from build123d import *

# Parameters (mm, degrees)
SKETCH_2_R          = 37.505158637
SKETCH_2_R_2        = 2.3
EXTRUDE_2_DEPTH     = 8
SKETCH_3_R          = 33
CUT_EXTRUDE_1_DEPTH = 5
CUT_EXTRUDE_START   = -16
SKETCH_3_2_R        = 33
CUT_EXTRUDE_2_DEPTH = 5


with BuildPart() as part:
    # Sketch 1 → Revolve 1 (revolve)
    with BuildSketch(Plane(origin=(0, 0, 0), x_dir=(0, 0, -1), z_dir=(1, 0, 0))):
        with BuildLine():
            Line((-8, 37.505158637), (8, 37.505158637))
            Line((8, 37.505158637), (10, 41.082575695))
            ThreePointArc((10, 41.082575695), (0, 47.5), (-10, 41.082575695))
            Line((-10, 41.082575695), (-8, 37.505158637))
        make_face()
    revolve(axis=Axis((0, 0, 15.4), (0, 0, -1)))

    # Sketch 2 → Extrude 2 (add, symmetric)
    with BuildSketch(Plane.XY):
        Circle(SKETCH_2_R)
        Circle(SKETCH_2_R_2, mode=Mode.SUBTRACT)
        with Locations((0, 8)):
            Circle(SKETCH_2_R_2, mode=Mode.SUBTRACT)
        with Locations((6.92820323, 4)):
            Circle(SKETCH_2_R_2, mode=Mode.SUBTRACT)
        with Locations((6.92820323, -4)):
            Circle(SKETCH_2_R_2, mode=Mode.SUBTRACT)
        with Locations((0, -8)):
            Circle(SKETCH_2_R_2, mode=Mode.SUBTRACT)
        with Locations((-6.92820323, -4)):
            Circle(SKETCH_2_R_2, mode=Mode.SUBTRACT)
        with Locations((-6.92820323, 4)):
            Circle(SKETCH_2_R_2, mode=Mode.SUBTRACT)
        with BuildLine():
            Line((5, 30.594117082), (5, 8.660254038))
            Line((5, 8.660254038), (23.995282599, 19.62718556))
            ThreePointArc((23.995282599, 19.62718556), (15.5, 26.846787517), (5, 30.594117082))
        make_face(mode=Mode.SUBTRACT)
        with BuildLine():
            Line((10, 0), (28.995282599, -10.966931522))
            ThreePointArc((28.995282599, -10.966931522), (31, 0), (28.995282599, 10.966931522))
            Line((28.995282599, 10.966931522), (10, 0))
        make_face(mode=Mode.SUBTRACT)
        with BuildLine():
            Line((5, -8.660254038), (5, -30.594117082))
            ThreePointArc((5, -30.594117082), (15.5, -26.846787517), (23.995282599, -19.62718556))
            Line((23.995282599, -19.62718556), (5, -8.660254038))
        make_face(mode=Mode.SUBTRACT)
        with BuildLine():
            Line((-5, -8.660254038), (-23.995282599, -19.62718556))
            ThreePointArc((-23.995282599, -19.62718556), (-15.5, -26.846787517), (-5, -30.594117082))
            Line((-5, -30.594117082), (-5, -8.660254038))
        make_face(mode=Mode.SUBTRACT)
        with BuildLine():
            Line((-10, 0), (-28.995282599, 10.966931522))
            ThreePointArc((-28.995282599, 10.966931522), (-31, 0), (-28.995282599, -10.966931522))
            Line((-28.995282599, -10.966931522), (-10, 0))
        make_face(mode=Mode.SUBTRACT)
        with BuildLine():
            Line((-5, 8.660254038), (-5, 30.594117082))
            ThreePointArc((-5, 30.594117082), (-15.5, 26.846787517), (-23.995282599, 19.62718556))
            Line((-23.995282599, 19.62718556), (-5, 8.660254038))
        make_face(mode=Mode.SUBTRACT)
        with BuildLine():
            Line((-2.90470199, 30.863614603), (-2.90470199, 11.729037589))
            Line((-2.90470199, 11.729037589), (2.90470199, 11.729037589))
            Line((2.90470199, 11.729037589), (2.90470199, 30.863614603))
            ThreePointArc((2.90470199, 30.863614603), (0, 31), (-2.90470199, 30.863614603))
        make_face(mode=Mode.SUBTRACT)
        with BuildLine():
            Line((8.705293519, 8.380064508), (11.609995509, 3.34897308))
            Line((11.609995509, 3.34897308), (28.181025294, 12.916261587))
            ThreePointArc((28.181025294, 12.916261587), (26.846787517, 15.5), (25.276323303, 17.947353015))
            Line((25.276323303, 17.947353015), (8.705293519, 8.380064508))
        make_face(mode=Mode.SUBTRACT)
        with BuildLine():
            Line((11.609995509, -3.34897308), (8.705293519, -8.380064508))
            Line((8.705293519, -8.380064508), (25.276323303, -17.947353015))
            ThreePointArc((25.276323303, -17.947353015), (26.846787517, -15.5), (28.181025294, -12.916261587))
            Line((28.181025294, -12.916261587), (11.609995509, -3.34897308))
        make_face(mode=Mode.SUBTRACT)
        with BuildLine():
            Line((2.90470199, -11.729037589), (-2.90470199, -11.729037589))
            Line((-2.90470199, -11.729037589), (-2.90470199, -30.863614603))
            ThreePointArc((-2.90470199, -30.863614603), (0, -31), (2.90470199, -30.863614603))
            Line((2.90470199, -30.863614603), (2.90470199, -11.729037589))
        make_face(mode=Mode.SUBTRACT)
        with BuildLine():
            Line((-8.705293519, -8.380064508), (-11.609995509, -3.34897308))
            Line((-11.609995509, -3.34897308), (-28.181025294, -12.916261587))
            ThreePointArc((-28.181025294, -12.916261587), (-26.846787517, -15.5), (-25.276323303, -17.947353015))
            Line((-25.276323303, -17.947353015), (-8.705293519, -8.380064508))
        make_face(mode=Mode.SUBTRACT)
        with BuildLine():
            Line((-11.609995509, 3.34897308), (-8.705293519, 8.380064508))
            Line((-8.705293519, 8.380064508), (-25.276323303, 17.947353015))
            ThreePointArc((-25.276323303, 17.947353015), (-26.846787517, 15.5), (-28.181025294, 12.916261587))
            Line((-28.181025294, 12.916261587), (-11.609995509, 3.34897308))
        make_face(mode=Mode.SUBTRACT)
    extrude(amount=EXTRUDE_2_DEPTH, both=True)

    # Sketch 3 → Cut-Extrude 1 (cut)
    with BuildSketch(Plane.XY.offset(8)):
        Circle(SKETCH_3_R)
    extrude(amount=-CUT_EXTRUDE_1_DEPTH, mode=Mode.SUBTRACT)

    # Sketch 3_2 → Cut-Extrude 2 (cut)
    with BuildSketch(Plane.XY.offset(8).offset(CUT_EXTRUDE_START)):
        Circle(SKETCH_3_2_R)
    extrude(amount=CUT_EXTRUDE_2_DEPTH, mode=Mode.SUBTRACT)


solid = part.part
CAD build for the part. Positions are in the model's coordinates, mm. A direction names the side the tool comes from. Round coordinates to 2 decimals unless told otherwise and drop trailing zeros. Loops run counter-clockwise (first coordinate to the right, second up) from the corner with the lowest first, then second, coordinate; pieces in that order, holes last.
(1) Drop flat-ended pins along their axis: pin 1 (5 mm diameter, centred on y = 18, z = -4, fed in from -X); pin 2 (5 mm diameter, centred on y = 21.5, z = 0, fed in from -X); pin 3 (7.5 mm diameter, centred on x = 0, y = -8, fed in from +Z). Give the stop position or say it passes through.
(2) Cut at B-B (z = -6.25). Give the cut face in (x, y).
(3) Which spindle directions (+Z, -Z, +X, -X, +Y, -Y) get a long thin tool onto all of the face, cutting with end or side? Do faces 1 (the flat face through (19.78, 8.066, 0.042)), 2 (the cylindrical face through (30.5, -12.6, 5.5)). Say none if no direction does.
(4) Cut at D-D (z = 5.75). Give the cut face in (x, y) (1 decimal), plus the area to 3 significant figures.
(5) Cut at A-A (x = 0). State how many separate pieces and enclosed holes the cut face has, plus the area to 3 significant figures.
(6) Wall check: line 1 along X through (y, z) = (-8.5, -1.75) (3 decimals); line 2 along Y through (x, z) = (-25.5, 8.5); line 3 along Y through (x, z) = (-1, 0.5). Give the ranges that are in metal, low to high.
Findings below:
1. pin 1: stops at x = -44.42
1. pin 2: stops at x = -43.53
1. pin 3: stops at z = 3
2. outline: circle Ø91.1 at (0, 0); hole circle Ø66 at (0, 0)
3. face 1: +Z, -Z
3. face 2: +Z
4. outline: circle Ø91.8 at (0, 0); hole circle Ø66 at (0, 0)
4. area: 3,190 mm2
5. separate pieces: 6
5. enclosed holes: 0
5. area: 539 mm2
6. line 1: x = -46.591 to -29.812, -24.722 to -20.532, -8.913 to -2.245, 2.245 to 8.913, 20.532 to 24.722, 29.812 to 46.591
6. line 2: y = -35.22 to -28.71, 28.71 to 35.22
6. line 3: y = -47.48 to -30.98, -11.73 to -10.07, -5.93 to -2.07, 2.07 to 5.93, 10.07 to 11.73, 30.98 to 47.48
